```python
from build123d import *

# Parameters (mm, degrees)
SKETCH1_R           = 2
BOSS_EXTRUDE1_DEPTH = 22
CUT_EXTRUDE1_DEPTH  = 6.5
CUT_EXTRUDE3_DEPTH  = 9.8
FILLET2_R           = 3
SKETCH7_R           = 1.6
CUT_EXTRUDE4_DEPTH  = 62.243285382
SKETCH8_R           = 3
CUT_EXTRUDE5_DEPTH  = 54.839948035
BOSS_EXTRUDE3_DEPTH = 22


with BuildPart() as part:
    # Sketch1 → Boss-Extrude1 (new body)
    with BuildSketch(Plane(origin=(0, 0, 0), x_dir=(1, 0, 0), z_dir=(0, 1, 0))):
        with BuildLine():
            Line((-39.3, 28.5), (-39.3, -6.5))
            Line((-39.3, -6.5), (0, -6.5))
            ThreePointArc((0, -6.5), (6.5, 0), (0, 6.5))
            ThreePointArc((0, 6.5), (-17.72074287, 12.087328765), (-26.300362263, 28.568624275))
            ThreePointArc((-26.300362263, 28.568624275), (-32.834312616, 34.999909434), (-39.3, 28.5))
        make_face()
        with Locations(Location((0, 0, 0), (0, 0, 270))):
            Circle(SKETCH1_R, mode=Mode.SUBTRACT)
        with Locations(Location((-32.8, 28.5, 0), (0, 0, 270))):
            Circle(SKETCH1_R, mode=Mode.SUBTRACT)
    extrude(amount=BOSS_EXTRUDE1_DEPTH)

    # Sketch2 → Cut-Extrude1 (cut)
    with BuildSketch(Plane.XY.offset(6.5)):
        Polygon((-17.1, 2.3), (-28.1, 2.3), (-28.1, 5.3), (-30.082842712, 5.3), (-33.082842712, 2.3), (-39.3, 2.3), (-39.3, 0), (-17.1, 0), align=None)
        Polygon((-39.5, 19.7), (-33.082842712, 19.7), (-30.082842712, 16.7), (-20.217157288, 16.7), (-17.100012785, 19.817144502), (-17.099645022, 22.2), (-39.5, 22.2), align=None)
    extrude(amount=-CUT_EXTRUDE1_DEPTH, mode=Mode.SUBTRACT)

    # Sketch6 → Cut-Extrude3 (cut)
    with BuildSketch(Plane.XZ):
        with BuildLine():
            Line((-6.5, 6.5), (0, 6.5))
            ThreePointArc((0, 6.5), (6.5, 0), (0, -6.5))
            ThreePointArc((0, -6.5), (-7.470973074, -7.005610766), (-14.432472984, -9.763979833))
            Line((-14.432472984, -9.763979833), (-6.5, 6.5))
        make_face()
    extrude(amount=-CUT_EXTRUDE3_DEPTH, mode=Mode.SUBTRACT)

    # Fillet2
    fillet2_edges = [part.edges().sort_by_distance(p)[0] for p in [
        (-10.466236492, 9.8, -1.631989916),
        (-10.466236492, 0, -1.631989916),
    ]]
    fillet(fillet2_edges, radius=FILLET2_R)

    # Sketch7 → Cut-Extrude4 (cut, through all)
    with BuildSketch(Plane.XY.offset(6.5)):
        with Locations((-22, 9.3)):
            Circle(SKETCH7_R)
    extrude(amount=-CUT_EXTRUDE4_DEPTH, mode=Mode.SUBTRACT)

    # Sketch8 → Cut-Extrude5 (cut, through all)
    with BuildSketch(Plane.XY.offset(-5.5)):
        with Locations((-22, 9.3)):
            Circle(SKETCH8_R)
    extrude(amount=-CUT_EXTRUDE5_DEPTH, mode=Mode.SUBTRACT)

    # Sketch9 → Boss-Extrude3 (add)
    with BuildSketch(Plane(origin=(0, 22, 0), x_dir=(1, 0, 0), z_dir=(0, 1, 0))):
        Polygon((-39.3, 8.575003739), (-47.980351229, 8.575003739), (-60.69390833, 1.234828124), (-63.156406461, 5.5), (-49.3, 13.5), (-39.3, 13.5), align=None)
    extrude(amount=-BOSS_EXTRUDE3_DEPTH)


solid = part.part
```
Can you work these out from the model? Positions are in its coordinate system, mm. A direction names the side the tool comes from. Coordinates: 2 decimals unless noted, no trailing zeros. Write each loop counter-clockwise with the first axis right and the second up, starting at its lowest first coordinate (ties: lowest second). Pieces come first, ordered by that corner, then holes. Notation, with made-up numbers: M -34,35 L 11,35 A18 ccw 11,60 Z; hole C 87,85.25 d10. An arc over 180 degrees is marked long. Answer as CSV lines item,"result".
Item 1: I'm going to push flat-ended pins straight in: P1, Ø5, axis at x = -45.5, y = 9.5, coming from the -Z side; P2, Ø8, axis at y = 19.5, z = -19.5, coming from the -X side; P3, Ø10, axis at x = -46.5, z = 1, coming from the -Y side; P4, Ø4.5, axis at x = -44, y = 9.5, coming from the +Z side (3 decimals). Where does each tip first touch, or does it pass through?
Geometry results:
P1,"stops at z = -13.5"
P2,"stops at x = -39.3"
P3,"passes through"
P4,"stops at z = -8.575"
Item 2: Imagine slicing it at B-B on x = -22. List the corners of the cut face in (y, z) for me.
Geometry results:
outline,"M 0,-16.76 L 6.3,-16.76 L 6.3,-5.5 L 7.7,-5.5 L 7.7,6.5 L 2.3,6.5 L 2.3,0 L 0,0 Z; M 10.9,-5.5 L 12.3,-5.5 L 12.3,-16.76 L 22,-16.76 L 22,0 L 16.7,0 L 16.7,6.5 L 10.9,6.5 Z"
Item 3: We'd pull the mould along X, two halves only. Please class faces 1 (the flat face through (-29, 22, -10)), 2 (the cylindrical face through (-32.199, 10.846, -26.592)), 3 (the flat face through (-61.91, 11.15, -3.34)): +X half, -X half, draft (parallel to the pull), parting line (faces both ways), or undercut.
Geometry results:
face 1,"draft"
face 2,"undercut"
face 3,"-X half"
Item 4: On a 3-axis mill with a long thin cutter (end or side, diameter ignored), from which of +Z, -Z, +X, -X, +Y, -Y can I reach the whole of each face in a straight line? I mean faces 4 (the flat face through (-18.68, 18.237, 3.296)), 5 (the flat face through (-28.1, 4, 3)), 6 (the flat face through (-44, 11, -13.5)), 7 (the flat face through (-44, 11, -8.575)), 8 (the flat face through (-10.5, 4.9, -1.7)). Say none if no direction works.
Geometry results:
face 4,"+Z, +Y"
face 5,"+Z, -Y"
face 6,"-Z, -X, +Y, -Y"
face 7,"+Z, +Y, -Y"
face 8,"-Z, +X, -Y"
Item 5: Imagine slicing it at C-C on z = -4. State how many separate pieces and enclosed holes the cut face has, plus the area to 3 significant figures.
Geometry results:
separate pieces,"2"
enclosed holes,"1"
area,"946 mm2"
Item 6: Imagine slicing it at D-D on x = -46.5. List the corners of the cut face in (y, z) for me (3 decimals), plus the area to 3 significant figures.
Geometry results:
outline,"M 0,-13.5 L 22,-13.5 L 22,-8.575 L 0,-8.575 Z"
area,"108 mm2"
Item 7: Please list where these lines run through material, in increasing order: line 1 along Y through (x, z) = (-22, 0.5); line 2 along Y through (x, z) = (-22, -9.75); line 3 along X through (y, z) = (8.5, -28.5).
Geometry results:
line 1,"y = 2.3 to 7.7, 10.9 to 16.7"
line 2,"y = 0 to 6.3, 12.3 to 22"
line 3,"x = -39.3 to -34.8, -30.8 to -26.29"
Item 8: Imagine slicing it at A-A on z = -29.5. List the corners of the cut face in (x, y) for me, plus the area to 3 significant figures.
Geometry results:
outline,"M -39.22,0 L -34.53,0 L -34.53,22 L -39.22,22 Z; M -31.07,0 L -26.38,0 L -26.38,22 L -31.07,22 Z"
area,"206 mm2"
